Check sheet for the modelled part. Datum: model origin and axes. Units: mm. Coordinates: 2 decimals unless noted, no trailing zeros. Write each loop counter-clockwise with the first axis right and the second up, starting at its lowest first coordinate (ties: lowest second). Pieces come first, ordered by that corner, then holes. Notation, with made-up numbers: M 33.5,39.5 L 43.5,39.5 A25 ccw 43.5,63.5 Z; hole C 35.25,-33 d10. An arc over 180 degrees is marked long. Answer as CSV lines item,"result". Start each with the question number.
Q1. Thickness scan on line 1 along X through (y, z) = (266, 52); line 2 along X through (y, z) = (283, -7.5); line 3 along Y through (x, z) = (-768.5, -64). Record the ranges inside material, lowest first. Write a range as from..to.
Q2. Sectioned sample at B-B, the plane x = -939.5. Record the cut outline in (y, z), then the cut area to 3 significant figures.
Q3. Sectioned sample at A-A, the plane y = 360. Record the cut outline in (x, z).
Q4. Mould release check, pull along Y, two halves, no side actions. Record for faces 1 (the flat face through (-18, -676.22, 2)), 2 (the flat face through (-1270, -9, 2)), 3 (the cylindrical face through (-973.416, 268.06, 1.778)): pulls with the +Y half, pulls with the -Y half, needs draft (parallel to the pull), parting line crosses it, or undercut.
Q5. Sectioned sample at C-C, the plane z = -76. Record the cut outline in (x, y), then the cut area to 3 significant figures.
from build123d import *

# Parameters (mm, degrees)
F0_W     = 2540
F0_H     = 1352.439214
F1_DEPTH = 127
F2_R     = 243.256461
F3_DEPTH = 254.001


with BuildPart() as f1:
    # F0 (on Top) → F1 (new body, symmetric)
    with BuildSketch(Plane.XY):
        Rectangle(F0_W, F0_H)
    extrude(amount=F1_DEPTH, both=True)

    # F2 (on face) → F3 (cut, through all)
    with BuildSketch(Plane.XY.offset(127)):
        with Locations((-730.394423, 257.364362)):
            Circle(F2_R)
    extrude(amount=-F3_DEPTH, mode=Mode.SUBTRACT)


solid = f1.part
Output:
1,line 1,"x = -1270..-973.5, -487.29..1270"
1,line 2,"x = -1270..-972.3, -488.49..1270"
1,line 3,"y = -676.22..17.11, 497.62..676.22"
2,outline,"M -676.22,-127 L 133.07,-127 L 133.07,127 L -676.22,127 Z; M 381.66,-127 L 676.22,-127 L 676.22,127 L 381.66,127 Z"
2,area,"280,000 mm^2"
3,outline,"M -1270,-127 L -950.94,-127 L -950.94,127 L -1270,127 Z; M -509.85,-127 L 1270,-127 L 1270,127 L -509.85,127 Z"
4,face 1,"pulls with the -Y half"
4,face 2,"needs draft"
4,face 3,"undercut"
5,outline,"M -1270,-676.22 L 1270,-676.22 L 1270,676.22 L -1270,676.22 Z; hole C -730.39,257.36 d486.51"
5,area,"3,250,000 mm^2"
